Study the drawing (mm; zero at the part's minimum x, y, z) and answer. Coordinates: 2 decimals unless noted, no trailing zeros. Write each loop counter-clockwise with the first axis right and the second up, starting at its lowest first coordinate (ties: lowest second). Pieces come first, ordered by that corner, then holes. Notation, with made-up numbers: M 48,-18.5 L 68,-18.5 A24 cw 68,-1.5 Z; hole C 81.25,-13 d2. An arc over 180 degrees is marked long. Answer as CSV lines item,"result". Start each with the question number.
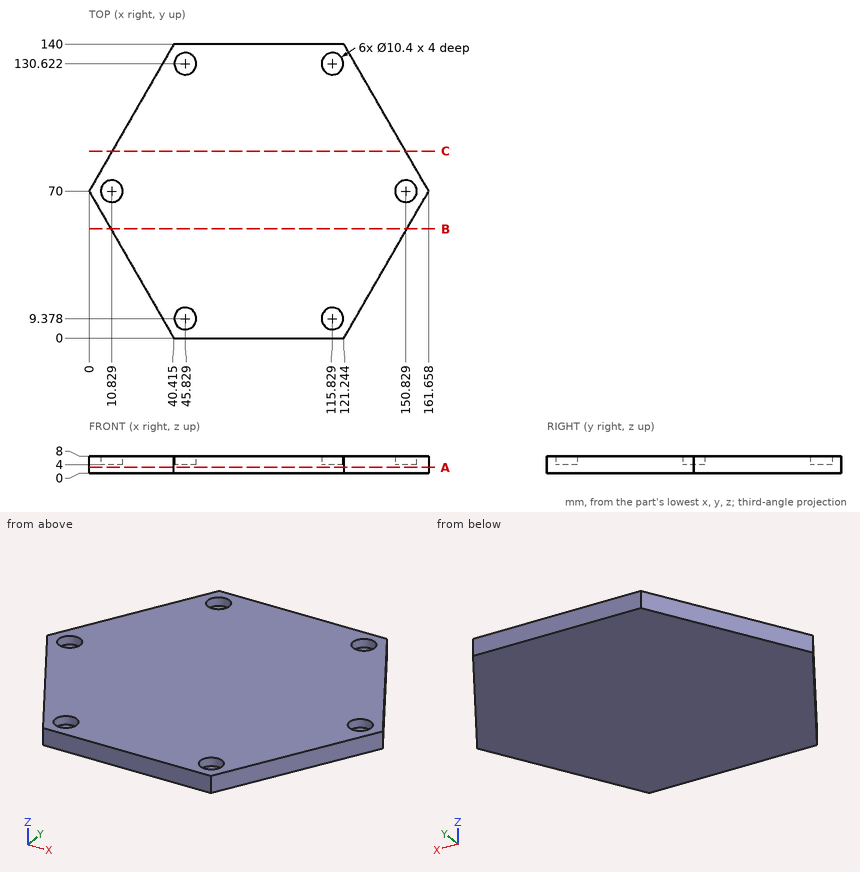
1) The part is cut by section A-A (z = 2.75). Determine the outline of the cut face in (x, y) (1 decimal).
2) Find the intervals of material crossed by line 1 (X direction, y = 72, z = 5.25) (1 decimal); line 2 (X direction, y = 84.5, z = 3.25) (1 decimal); line 3 (Y direction, x = 25, z = 7.5) (1 decimal), in increasing order. Write a range as from..to.
3) Each of these flat-tipped pins is pushed along its axis until it touches: P1, Ø8.5, axis at x = 10.83, y = 70, coming from the +Z side; P2, Ø3, axis at y = 63, z = 6.5, coming from the -X side (1 decimal); P3, Ø1.5, axis at y = 22.5, z = 5, coming from the -X side. Where does it stop, or does it pass through?
4) The part is cut by section C-C (y = 89). Determine the outline of the cut face in (x, z).
5) The part is cut by section B-B (y = 52). Determine the outline of the cut face in (x, z) (1 decimal), then the cut area to 3 significant figures.
Completed:
1,outline,"M 0,70 L 40.4,0 L 121.2,0 L 161.7,70 L 121.2,140 L 40.4,140 Z"
2,line 1,"1.2..6, 15.6..146, 155.6..160.5"
2,line 2,"8.4..153.3"
2,line 3,"26.7..113.3"
3,P1,"z = 4"
3,P2,"x = 3.2"
3,P3,"x = 26.99"
4,outline,"M 10.97,0 L 150.69,0 L 150.69,8 L 10.97,8 Z"
5,outline,"M 10.4,0 L 151.3,0 L 151.3,8 L 10.4,8 Z"
5,area,"1,130 mm²"
